Geometry check sheet. Reference: drawing and pictorial views, mm from the part's lowest x, y, z. Give positions to 0.01 mm unless a question says otherwise; leave off trailing zeros. Order: outer loops, then holes, each group sorted by start corner. A loop starts at its lowest first (then second) coordinate and runs counter-clockwise, first axis right, second up.
Item 1: Sectioned sample at C-C on z = 30. Record the boundary of the cut face in (x, y) (1 decimal).
Item 2: Material ranges on line 1 along X through (y, z) = (1.25, 35); line 2 along X through (y, z) = (1.15, 30) (1 decimal); line 3 along Z through (x, y) = (120, 0.55), recorded low to high.
Item 3: Sectioned sample at A-A on z = 15. Record the boundary of the cut face in (x, y).
Item 4: Sectioned sample at B-B on x = 72.5. Record the boundary of the cut face in (y, z), and give its area (3 significant figures).
Item 5: Gauge pin test, flat ends, axial feed: P1, Ø0.6, axis at x = 63, y = 1, coming from the -Z side; P2, Ø1.5, axis at x = 108.5, z = 29, coming from the -Y side. Record the tip position at first contact, or that the pin passes through.
Item 6: Sectioned sample at D-D on x = 120. Record the boundary of the cut face in (y, z), and give its area (3 significant figures).
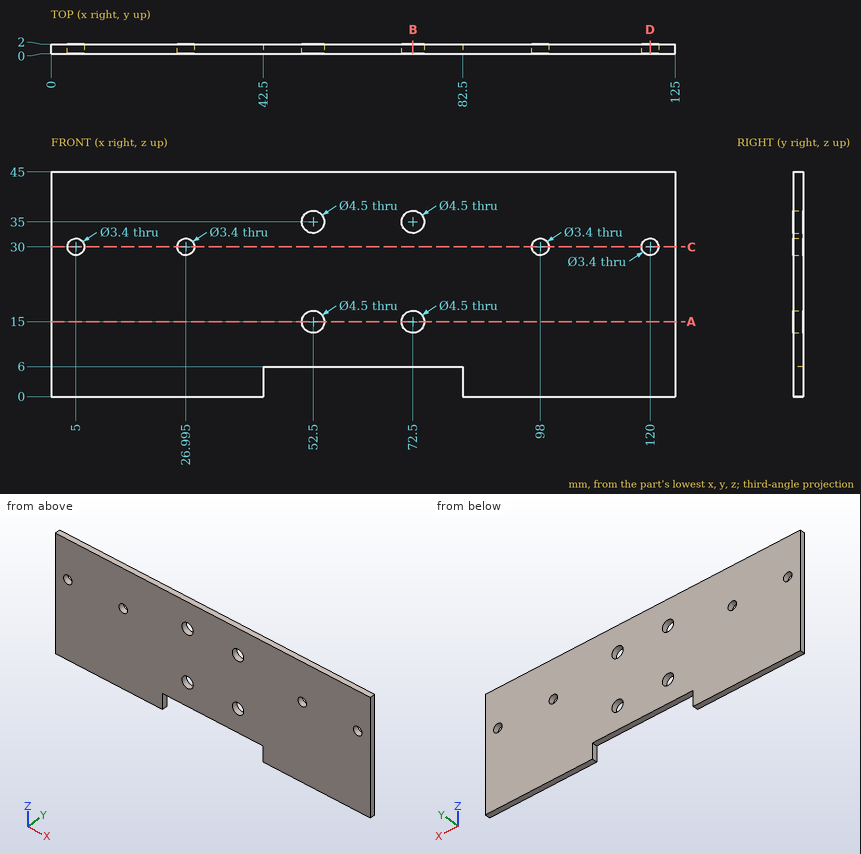
Report:
1. outline: (0, 0) - (3.3, 0) - (3.3, 2) - (0, 2) - close; (6.7, 0) - (25.3, 0) - (25.3, 2) - (6.7, 2) - close; (28.7, 0) - (96.3, 0) - (96.3, 2) - (28.7, 2) - close; (99.7, 0) - (118.3, 0) - (118.3, 2) - (99.7, 2) - close; (121.7, 0) - (125, 0) - (125, 2) - (121.7, 2) - close
2. line 1: x = 0 to 50.25, 54.75 to 70.25, 74.75 to 125
2. line 2: x = 0 to 3.3, 6.7 to 25.3, 28.7 to 96.3, 99.7 to 118.3, 121.7 to 125
2. line 3: z = 0 to 28.3, 31.7 to 45
3. outline: (0, 0) - (50.25, 0) - (50.25, 2) - (0, 2) - close; (54.75, 0) - (70.25, 0) - (70.25, 2) - (54.75, 2) - close; (74.75, 0) - (125, 0) - (125, 2) - (74.75, 2) - close
4. outline: (0, 6) - (2, 6) - (2, 12.75) - (0, 12.75) - close; (0, 17.25) - (2, 17.25) - (2, 32.75) - (0, 32.75) - close; (0, 37.25) - (2, 37.25) - (2, 45) - (0, 45) - close
4. area: 60.0 mm2
5. P1: stops at z = 6
5. P2: stops at y = 0
6. outline: (0, 0) - (2, 0) - (2, 28.3) - (0, 28.3) - close; (0, 31.7) - (2, 31.7) - (2, 45) - (0, 45) - close
6. area: 83.2 mm2
